The listing builds one solid part. Answer for the finished solid, in the listing's coordinates (mm). A direction names the side the tool comes from. Give positions to 0.01 mm unless a question says otherwise; leave off trailing zeros. Write each loop counter-clockwise with the first axis right and the second up, starting at its lowest first coordinate (ties: lowest second). Pieces come first, ordered by that corner, then holes. Notation, with made-up numbers: (76.5, 39.25) - (112.5, 39.25) arc R24 cw to (112.5, 58.25) - close; hole circle Ø1 at (28, 39). An arc over 180 degrees is marked (long way). Write each question's results on one line, items separated by ' | '. Start each with the question number.
Q1. Section B-B (y = 2.75) is taken. Determine the outline of the cut face in (x, z) (3 decimals).
Q2. Find the intervals of material crossed by probe 1 along X at (y, z) = (1.75, 0); probe 2 along X at (y, z) = (3.75, -1.25); probe 3 along Z at (x, y) = (0, 6.2), in increasing order.
Q3. Section C-C (y = 5.75) is taken. Determine the outline of the cut face in (x, z).
Q4. For a pull along X with two mould halves and no side action, classify faces 1 (the face through (28, 5, -5)), 2 (the face through (33.751, 2.465, -3.977)), 3 (the face through (54.47, 2.46, -11.41)) as pulls with the +X half, pulls with the -X half, needs draft (parallel to the pull), parting line crosses it, or undercut.
Q5. Section D-D (x = 10) is taken. Determine the outline of the cut face in (y, z), plus the area to 3 significant figures.
Q6. For faces 4 (the face through (44.583, 2.465, -6.107)), 5 (the face through (-4.88, 4.23, 1.08)), 6 (the face through (10, 2, -5)), determine the directions among +Z, -Z, +X, -X, +Y, -Y from which every point of the face is accessible in a straight line to the end or side of a thin tool.
Q7. Section A-A (z = 0) is taken. Determine the outline of the cut face in (x, y), plus the area to 3 significant figures.
Q8. Flat-ended cylindrical pins translate along their axes: pin 1 Ø1.8 at (x, z) = (22, 0) entering from +Y; pin 2 Ø1.5 at (x, y) = (3.5, 3.5) entering from -Z; pin 3 Ø2 at (x, y) = (28, 3) entering from -Z; pin 4 Ø1.5 at (y, z) = (1.5, 1) entering from +X. Find the tip coordinate at first contact, or state that the pin passes through.
Autodesk Fusion 360 part; units mm, degrees
sketch "Sketch1" plane through (0, 0, 0) normal (0, 1, 0) x (1, 0, 0)
  line L0 (0, -5) -> (22, -5)
  arc A0 (22, -5) -> (22, 5) centre (22, 0) ccw
  line L1 (22, 5) -> (0, 5)
  arc A1 (0, 5) -> (0, -5) centre (0, 0) ccw
  line L2 (0, 0) -> (22, 0) construction
  circle A2 centre (0, 0) radius 1.5
  line L3 (20.35, 5) -> (51.8071, 17.9015)
  line L4 (51.8071, 17.9015) -> (55.6974, 8.4161)
  line L5 (55.6974, 8.4161) -> (23.8973, -4.626)
  line L6 (46.255, 15.6244) -> (53.278, 14.3153)
  line L7 (48.6059, 5.5077) -> (40.4462, 6.7233)
  line L8 (40.4462, 6.7233) -> (26.8652, 1.1533)
  circle A3 centre (22, 0) radius 1.5
  dimension "d1" = 22
  dimension "d3" = 5
  dimension "d4" = 3
  dimension "d5" = 157.7
  dimension "d6" = 34
  dimension "d7" = 1.65
  dimension "d8" = 3
extrude "Extrude1" add sketch "Sketch1" along normal blind 5 contours L0 A0 L1 A1 | A0 L1 L3 L4 L5 L6 L7 L8
sketch "Sketch2" plane through (0, 0, 0) normal (0, 1, 0) x (1, 0, 0)
sketch "Sketch3" plane through (0, 5, 0) normal (0, 1, 0) x (-1, 0, 0)
  circle A0 centre (0, 0) radius 1.5
  circle A1 centre (-22, 0) radius 1.5
  line L0 (-20.35, -5) -> (0, -5)
  arc A2 (0, -5) -> (0, 5) centre (0, 0) ccw
  line L1 (0, 5) -> (-22, 5)
  arc A3 (-22, 5) -> (-26.8652, -1.1533) centre (-22, 0) ccw
  line L2 (-26.8652, -1.1533) -> (-40.4462, -6.7233)
  line L3 (-40.4462, -6.7233) -> (-48.6059, -5.5077)
  line L4 (-48.6059, -5.5077) -> (-55.6974, -8.4161)
  line L5 (-55.6974, -8.4161) -> (-53.278, -14.3153)
  line L6 (-53.278, -14.3153) -> (-46.255, -15.6244)
  line L7 (-46.255, -15.6244) -> (-20.35, -5)
  circle A4 centre (0, 0) radius 5
  dimension "d11" = 10
extrude "Extrude2" add sketch "Sketch3" along normal blind 2 contours A2 A4
Answers below:
1) outline: (0, -5) - (20.35, -5) - (46.255, -15.624) - (53.278, -14.315) - (55.697, -8.416) - (48.606, -5.508) - (40.446, -6.723) - (26.865, -1.153) arc R5 ccw to (22, 5) - (0, 5) arc R5 ccw to start; hole circle Ø3 at (0, 0); hole circle Ø3 at (22, 0)
2) probe 1: x = -5 to -1.5, 1.5 to 20.5, 23.5 to 27 | probe 2: x = -4.84 to -0.83, 0.83 to 21.17, 22.83 to 27.1 | probe 3: z = -5 to -1.5, 1.5 to 5
3) outline: circle Ø10 at (0, 0); hole circle Ø3 at (0, 0)
4) face 1: needs draft | face 2: undercut | face 3: pulls with the +X half
5) outline: (0, -5) - (5, -5) - (5, 5) - (0, 5) - close | area: 50.0 mm2
6) face 4: +Z, +Y, -Y | face 5: +Y | face 6: -Z, -X, +Y, -Y
7) outline: (-5, 0) - (-1.5, 0) - (-1.5, 7) - (-5, 7) - close; (1.5, 0) - (20.5, 0) - (20.5, 5) - (5, 5) - (5, 7) - (1.5, 7) - close; (23.5, 0) - (27, 0) - (27, 5) - (23.5, 5) - close | area: 144 mm2
8) pin 1: passes through | pin 2: stops at z = -5 | pin 3: stops at z = -8.55 | pin 4: stops at x = 26.99
